from build123d import *

# Parameters (mm, degrees)
SKETCH_1_W          = 18
SKETCH_1_H          = 22
EXTRUDE_1_DEPTH     = 3.5
SKETCH_2_R          = 3.6
CUT_EXTRUDE_1_DEPTH = 3.5
SKETCH_3_R          = 5.525
CUT_EXTRUDE_2_DEPTH = 2.65
SKETCH_4_W          = 5
SKETCH_4_H          = 5
EXTRUDE_2_DEPTH     = 2
FILLET_1_RADIUS     = 2.5
FILLET_1_LENGTH     = 2
SKETCH_5_R          = 1.1
CUT_EXTRUDE_3_DEPTH = 3
SKETCH_6_W          = 18
SKETCH_6_H          = 3.5
EXTRUDE_3_DEPTH     = 1


with BuildPart() as part:
    # 草图1 → 凸台-拉伸1 (new body)
    with BuildSketch(Plane.XY):
        Rectangle(SKETCH_1_W, SKETCH_1_H)
    extrude(amount=EXTRUDE_1_DEPTH)

    # 草图2 → 切除-拉伸1 (cut)
    with BuildSketch(Plane.XY.offset(3.5)):
        with Locations((0, 3)):
            Circle(SKETCH_2_R)
    extrude(amount=-CUT_EXTRUDE_1_DEPTH, mode=Mode.SUBTRACT)

    # 草图3 → 切除-拉伸2 (cut)
    with BuildSketch(Plane.XY.offset(3.5)):
        with Locations((0, 3)):
            Circle(SKETCH_3_R)
    extrude(amount=-CUT_EXTRUDE_2_DEPTH, mode=Mode.SUBTRACT)

    # 草图4 → 凸台-拉伸2 (add)
    with BuildSketch(Plane.XZ.offset(11)):
        with Locations((-6.5, 6)):
            Rectangle(SKETCH_4_W, SKETCH_4_H)
    extrude(amount=-EXTRUDE_2_DEPTH)

    # 圆角1: full round fillet: the end face becomes a half cylinder, R = half its width
    fillet_1_face = Plane((-6.5, -10, 8.5), x_dir=(0, -1, 0), z_dir=(0, 0, 1))  # on the end face: x along it, z out of the body
    fillet_1_slab = fillet_1_face.offset(-FILLET_1_RADIUS / 2) * Box(FILLET_1_LENGTH, 2 * FILLET_1_RADIUS, FILLET_1_RADIUS, mode=Mode.PRIVATE)  # the body's end, R deep
    fillet_1_round = Plane((-6.5, -10, 6), x_dir=(0, 0, 1), z_dir=(0, -1, 0)) * Cylinder(FILLET_1_RADIUS, FILLET_1_LENGTH, mode=Mode.PRIVATE)  # its axis R under the face
    add(fillet_1_slab - fillet_1_round, mode=Mode.SUBTRACT)

    # 草图5 → 切除-拉伸3 (cut)
    with BuildSketch(Plane(origin=(0, -9, 0), x_dir=(1, 0, 0), z_dir=(0, 1, 0))):
        with Locations(Location((-6.5, -6, 0), (0, 0, 270))):
            Circle(SKETCH_5_R)
    extrude(amount=-CUT_EXTRUDE_3_DEPTH, mode=Mode.SUBTRACT)

    # 镜向6: part across plane


with BuildPart() as part_1:
    add(part.part)
    add(part.part.mirror(Plane.ZY))

    # 草图6 → 凸台-拉伸3 (add)
    with BuildSketch(Plane.XZ.offset(11)):
        with Locations((0, 1.75)):
            Rectangle(SKETCH_6_W, SKETCH_6_H)
    extrude(amount=EXTRUDE_3_DEPTH)


solid = part_1.part
Input: part model. Units: mm. Frame: model coordinates. A direction names the side the tool comes from. Give positions to 0.01 mm unless a question says otherwise; leave off trailing zeros. Order: outer loops, then holes, each group sorted by start corner. A loop starts at its lowest first (then second) coordinate and runs counter-clockwise, first axis right, second up.
Q1. Section C-C on y = 3. Output: boundary loops of the cut face in (x, z) (3 decimals), and give its area (3 significant figures).
Checked values:
outline: (-9, 0) - (-3.6, 0) - (-3.6, 0.85) - (-5.525, 0.85) - (-5.525, 3.5) - (-9, 3.5) - close; (3.6, 0) - (9, 0) - (9, 3.5) - (5.525, 3.5) - (5.525, 0.85) - (3.6, 0.85) - close
area: 27.6 mm2
Q2. Section A-A on z = 3. Output: boundary loops of the cut face in (x, y) (3 decimals), and give its area (3 significant figures).
Checked values:
outline: (-9, -12) - (9, -12) - (9, 11) - (-9, 11) - close; hole circle Ø11.05 at (0, 3)
area: 318 mm2
Q3. Contact query for flat-ended pins moving along their axis: pin 1 Ø4 at (x, y) = (-3.5, -6.5) entering from +Z; pin 2 Ø4 at (x, z) = (7.5, 5) entering from -Y; pin 3 Ø5.5 at (x, y) = (2.5, 2.5) entering from +Z; pin 4 Ø3 at (x, z) = (6.5, 6) entering from -Y. Output: stop coordinate, or through.
Checked values:
pin 1: stops at z = 3.5
pin 2: stops at y = -12
pin 3: stops at z = 0.85
pin 4: stops at y = -11
Q4. Set-up query: faces 1 (the flat face through (-7.1, -9, 4.9)), 2 (the flat face through (-5.9, -11, 4.9)), 3 (the flat face through (4, -10, 5)), 4 (the flat face through (0, -1, 0.85)). Return all of +Z, -Z, +X, -X, +Y, -Y with unobstructed straight access to the full face (end or side cutting, diameter ignored); none if empty.
Checked values:
face 1: +Z, +X, -X, +Y
face 2: +Z, +X, -X, -Y
face 3: +Z, +Y, -Y
face 4: +Z
Q5. Ray query, probe 1 along X at (y, z) = (-10.25, 6); probe 2 along X at (y, z) = (3, 1.8) (3 decimals); probe 3 along Y at (x, z) = (0, 0.2). Return the intervals inside material, ascending.
Checked values:
probe 1: x = -9 to -7.6, -5.4 to -4, 4 to 5.4, 7.6 to 9
probe 2: x = -9 to -5.525, 5.525 to 9
probe 3: y = -12 to -0.6, 6.6 to 11
Q6. Section B-B on x = 0. Output: boundary loops of the cut face in (y, z) (3 decimals).
Checked values:
outline: (-12, 0) - (-0.6, 0) - (-0.6, 0.85) - (-2.525, 0.85) - (-2.525, 3.5) - (-12, 3.5) - close; (6.6, 0) - (11, 0) - (11, 3.5) - (8.525, 3.5) - (8.525, 0.85) - (6.6, 0.85) - close
Q7. Section D-D on z = 5.25. Output: boundary loops of the cut face in (x, y).
Checked values:
outline: (-9, -11) - (-7.3, -11) - (-7.3, -9) - (-9, -9) - close; (-5.7, -11) - (-4, -11) - (-4, -9) - (-5.7, -9) - close; (4, -11) - (5.7, -11) - (5.7, -9) - (4, -9) - close; (7.3, -11) - (9, -11) - (9, -9) - (7.3, -9) - close
Q8. Draft query along X for faces 5 (the flat face through (-9, 0, 2)), 6 (the flat face through (-4, -10, 5)), 7 (the flat face through (7.1, -9, 4.9)), 8 (the cylindrical face through (6.4, -10, 8.5)). Return one class per face: +X half, -X half, draft (parallel to the pull), parting line (faces both ways), or undercut.
Checked values:
face 5: -X half
face 6: undercut
face 7: draft
face 8: undercut
